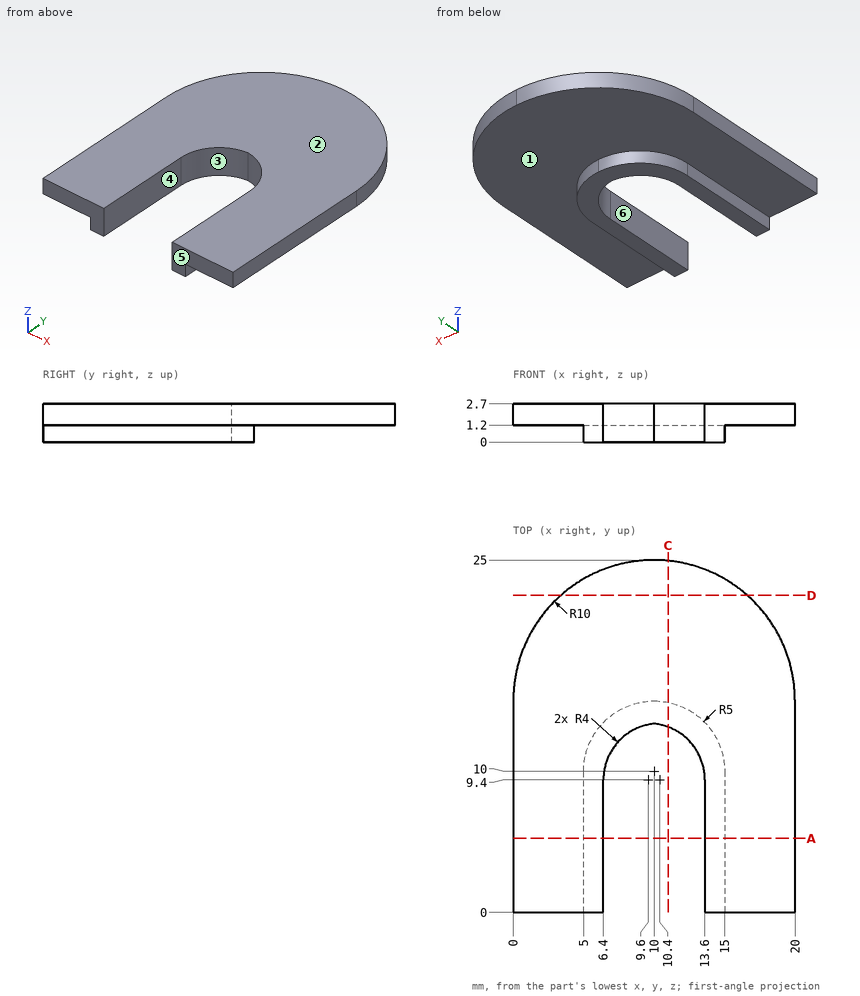
Check sheet for the drawn part. Datum: minimum x, y, z corner. Units: mm. A direction names the side the tool comes from. Round coordinates to 2 decimals unless told otherwise and drop trailing zeros. Loops run counter-clockwise (first coordinate to the right, second up) from the corner with the lowest first, then second, coordinate; pieces in that order, holes last. Notation, with made-up numbers: (-19.5, 71.5) -> (15.5, 71.5) arc R12 ccw to (15.5, 79.5) -> close; hole circle Ø5 at (51.5, 74). An arc over 180 degrees is marked (long way). Put each result on its own line as item: value. Start each with the question number.
1. Section check C-C (x = 11). Enter the section's corners in (y, z), plus the area to 3 significant figures.
2. Section check D-D (y = 22.5). Enter the section's corners in (x, z).
3. Scan lines: probe 1 along X at (y, z) = (4, 0.95); probe 2 along X at (y, z) = (8.25, 2); probe 3 along Z at (x, y) = (18.5, 4). Record each from-to range of solid material in increasing order.
4. Section check A-A (y = 5.25). Enter the section's corners in (x, z).
5. Access from +Z, -Z, +X, -X, +Y, -Y to the whole of each face (thin tool, end or side, straight path). Record for the marked faces 1, 2 and 3.
6. Gauge pin test, flat ends, axial feed: pin 1 (1.3 mm diameter, centred on y = 3.5, z = 0.5, fed in from +X); pin 2 (1 mm diameter, centred on y = 22, z = 1.5, fed in from -X); pin 3 (1 mm diameter, centred on y = 4.5, z = 0.5, fed in from -X). Record the tip position at first contact, or that the pin passes through.
7. Draft check along X on the marked faces 4, 5 and 6. Enter one of: +X half, -X half, draft (parallel to the pull), parting line (faces both ways), or undercut.
Findings:
1. outline: (13.15, 0) -> (14.9, 0) -> (14.9, 1.2) -> (24.95, 1.2) -> (24.95, 2.7) -> (13.15, 2.7) -> close
1. area: 19.8 mm^2
2. outline: (3.39, 1.2) -> (16.61, 1.2) -> (16.61, 2.7) -> (3.39, 2.7) -> close
3. probe 1: x = 5 to 6.4, 13.6 to 15
3. probe 2: x = 0 to 6.4, 13.6 to 20
3. probe 3: z = 1.2 to 2.7
4. outline: (0, 1.2) -> (5, 1.2) -> (5, 0) -> (6.4, 0) -> (6.4, 2.7) -> (0, 2.7) -> close; (13.6, 0) -> (15, 0) -> (15, 1.2) -> (20, 1.2) -> (20, 2.7) -> (13.6, 2.7) -> close
5. face 1: -Z, +Y
5. face 2: +Z, +X, -X, +Y, -Y
5. face 3: +Z, -Z, -Y
6. pin 1: stops at x = 15
6. pin 2: stops at x = 2.4
6. pin 3: stops at x = 5
7. face 4: undercut
7. face 5: draft
7. face 6: undercut
